Check sheet for the drawn part. Datum: minimum x, y, z corner. Units: mm. A direction names the side the tool comes from. Round coordinates to 2 decimals unless told otherwise and drop trailing zeros. Loops run counter-clockwise (first coordinate to the right, second up) from the corner with the lowest first, then second, coordinate; pieces in that order, holes last. Notation, with made-up numbers: (-9, -14) -> (27, -14) arc R24 ccw to (27, 21) -> close; hole circle Ø7 at (-14, 82.25). An arc over 180 degrees is marked (long way). Return JSON: item names as keys, results as strings.
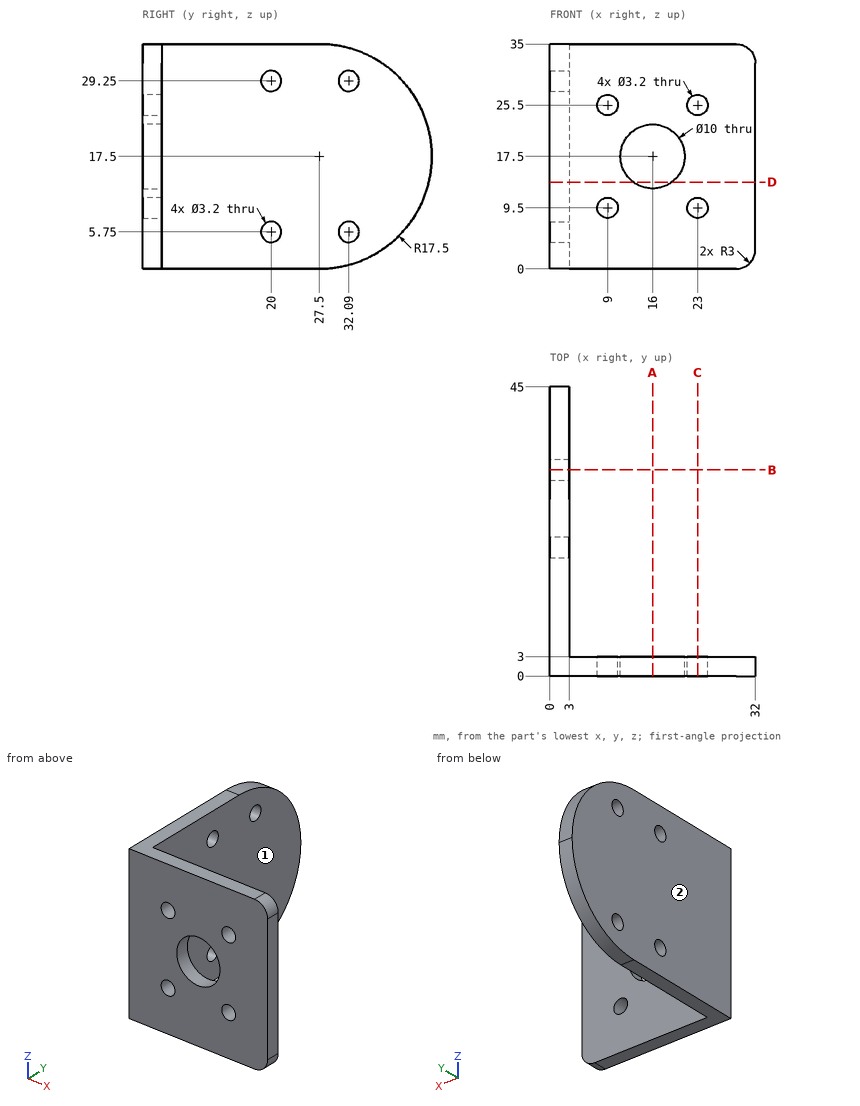
Q1. Material ranges on line 1 (Z direction, x = 1, y = 20); line 2 (X direction, y = 1.1, z = 9.5); line 3 (X direction, y = 5, z = 31), recorded low to high.
Results list:
{"line 1": "0 to 4.15, 7.35 to 27.65, 30.85 to 35", "line 2": "0 to 7.4, 10.6 to 21.4, 24.6 to 32", "line 3": "0 to 3"}
Q2. Go/stop test with flat-tipped pins: pin 1 (5 mm diameter, centred on y = 32.09, z = 5.75, fed in from +X); pin 2 (1.9 mm diameter, centred on x = 23, z = 9.5, fed in from +Y); pin 3 (4 mm diameter, centred on x = 9, z = 25.5, fed in from +Y). Record where each tip stops, or that it passes through.
Results list:
{"pin 1": "x = 3", "pin 2": "through", "pin 3": "y = 3"}
Q3. Section check D-D (z = 13.5). Record the boundary of the cut face in (x, y).
Results list:
{"outline": "(0, 0) -> (13, 0) -> (13, 3) -> (3, 3) -> (3, 44.54) -> (0, 44.54) -> close; (19, 0) -> (32, 0) -> (32, 3) -> (19, 3) -> close"}
Q4. Section check A-A (x = 16). Record the boundary of the cut face in (y, z).
Results list:
{"outline": "(0, 0) -> (3, 0) -> (3, 12.5) -> (0, 12.5) -> close; (0, 22.5) -> (3, 22.5) -> (3, 35) -> (0, 35) -> close"}
Q5. Section check C-C (x = 23). Record the boundary of the cut face in (y, z), then the cut area to 3 significant figures.
Results list:
{"outline": "(0, 0) -> (3, 0) -> (3, 7.9) -> (0, 7.9) -> close; (0, 11.1) -> (3, 11.1) -> (3, 23.9) -> (0, 23.9) -> close; (0, 27.1) -> (3, 27.1) -> (3, 35) -> (0, 35) -> close", "area": "85.8 mm^2"}
Q6. Section check B-B (y = 32.09). Record the boundary of the cut face in (x, z).
Results list:
{"outline": "(0, 0.61) -> (3, 0.61) -> (3, 4.15) -> (0, 4.15) -> close; (0, 7.35) -> (3, 7.35) -> (3, 27.65) -> (0, 27.65) -> close; (0, 30.85) -> (3, 30.85) -> (3, 34.39) -> (0, 34.39) -> close"}
Q7. Tool access check on the marked faces 1 and 2. Record the directions out of +Z, -Z, +X, -X, +Y, -Y that give a thin tool (end or side, any length) a straight path to the whole face; none if there is none.
Results list:
{"face 1": "+Z, -Z, +X, +Y", "face 2": "+Z, -Z, -X, +Y, -Y"}
